```python
from build123d import *

# Parameters (mm, degrees)
SKETCH1_W   = 14.0462
SKETCH1_H   = 10
SKETCH1_W_2 = 1.8288
SKETCH1_H_2 = 30.48


with BuildPart() as part:
    # Sketch1 → Revolve1 (revolve)
    with BuildSketch(Plane.XY, mode=Mode.PRIVATE) as revolve1_sk:
        with Locations((7.0231, 35.48)):
            Rectangle(SKETCH1_W, SKETCH1_H)
        Polygon((14.0462, 40.48), (14.0462, 30.48), (15.875, 30.48), (19.685, 30.48), (19.685, 65), (14.0462, 65), align=None)
        with Locations((14.9606, 15.24)):
            Rectangle(SKETCH1_W_2, SKETCH1_H_2)
    revolve(revolve1_sk.sketch.rotate(Axis((0, 0, 0), (0, 1, 0)), 90), axis=Axis((0, 0, 0), (0, 1, 0)))


solid = part.part
```
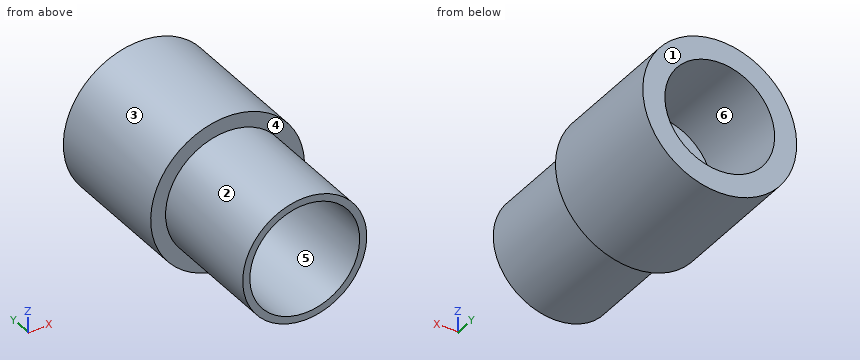
Check sheet for the modelled part. Datum: model origin and axes. Units: mm. Face numbers are marked on the shaded views. A direction names the side the tool comes from. Round coordinates to 2 decimals unless told otherwise and drop trailing zeros. Order: outer loops, then holes, each group sorted by start corner. A loop starts at its lowest first (then second) coordinate and runs counter-clockwise, first axis right, second up. Notation, with made-up numbers: (-40, 67) -> (-23, 67) arc R26 ccw to (-23, 94) -> close; hole circle Ø8 at (-33, -28.5). An arc over 180 degrees is marked (long way). One line per item, written item: value. Start each with the question number.
Q1. Thickness scan on line 1 (X direction, y = 56.25, z = 0) (3 decimals); line 2 (X direction, y = 17, z = 0) (3 decimals); line 3 (Y direction, x = -16.5, z = -1). Record the ranges inside material, lowest first.
Q2. Cross-section at C-C (y = 49). Record the boundary of the cut face in (x, z) (3 decimals).
Q3. Mould release check, pull along Z, two halves, no side actions. Record for the marked faces 3, 4, 5 and 6: pulls with the +Z half, pulls with the -Z half, needs draft (parallel to the pull), parting line crosses it, or undercut.
Q4. Set-up check for the marked faces 1 and 2: record each of +Z, -Z, +X, -X, +Y, -Y from which the full face is reachable in a straight line by a thin tool's end or side.
Q5. Cross-section at A-A (z = 0). Record the boundary of the cut face in (x, y) (3 decimals), and give its area (3 significant figures).
Q6. Gauge pin test, flat ends, axial feed: pin 1 Ø14 at (x, z) = (-5, -1.5) entering from -Y; pin 2 Ø3 at (x, y) = (-15.5, 50.5) entering from -Z; pin 3 Ø1 at (x, z) = (11, 6.5) entering from +Y. Record the tip position at first contact, or that the pin passes through.
Q7. Cross-section at D-D (x = 15). Record the boundary of the cut face in (y, z), and give its area (3 significant figures).
Q8. Cross-section at B-B (x = 0). Record the boundary of the cut face in (y, z) (3 decimals), and give its area (3 significant figures).
Completed:
1. line 1: x = -19.685 to -14.046, 14.046 to 19.685
1. line 2: x = -15.875 to -14.046, 14.046 to 15.875
1. line 3: y = 30.48 to 65
2. outline: circle Ø39.37 at (0, 0); hole circle Ø28.092 at (0, 0)
3. face 3: parting line crosses it
3. face 4: needs draft
3. face 5: undercut
3. face 6: undercut
4. face 1: +Z, -Z, +X, -X, +Y
4. face 2: -Y
5. outline: (-19.685, 30.48) -> (-15.875, 30.48) -> (-15.875, 0) -> (-14.046, 0) -> (-14.046, 30.48) -> (14.046, 30.48) -> (14.046, 0) -> (15.875, 0) -> (15.875, 30.48) -> (19.685, 30.48) -> (19.685, 65) -> (14.046, 65) -> (14.046, 40.48) -> (-14.046, 40.48) -> (-14.046, 65) -> (-19.685, 65) -> close
5. area: 782 mm²
6. pin 1: stops at y = 30.48
6. pin 2: stops at z = -13.84
6. pin 3: stops at y = 40.48
7. outline: (0, -5.2) -> (30.48, -5.2) -> (30.48, -12.75) -> (65, -12.75) -> (65, 12.75) -> (30.48, 12.75) -> (30.48, 5.2) -> (0, 5.2) -> close
7. area: 1,200 mm²
8. outline: (0, -15.875) -> (30.48, -15.875) -> (30.48, -19.685) -> (65, -19.685) -> (65, -14.046) -> (40.48, -14.046) -> (40.48, 14.046) -> (65, 14.046) -> (65, 19.685) -> (30.48, 19.685) -> (30.48, 15.875) -> (0, 15.875) -> (0, 14.046) -> (30.48, 14.046) -> (30.48, -14.046) -> (0, -14.046) -> close
8. area: 782 mm²
